The listing builds one solid part. Answer for the finished solid, in the listing's coordinates (mm). Round coordinates to 2 decimals unless told otherwise and drop trailing zeros. Order: outer loops, then holes, each group sorted by start corner. A loop starts at its lowest first (then second) coordinate and runs counter-clockwise, first axis right, second up. Notation, with made-up numbers: (-2, 81.25) -> (5, 81.25) arc R28 ccw to (5, 115.25) -> close; hole circle Ø4 at (38.25, 29). An arc over 180 degrees is marked (long way). Return JSON: item names as keys, results as strings. Group by question number.
(1) The part is cut by section D-D (x = -28.5). Determine the outline of the cut face in (y, z), plus the area to 3 significant figures.
(2) The part is cut by section A-A (y = 0). Determine the outline of the cut face in (x, z) (3 decimals), plus the area to 3 significant figures.
(3) The part is cut by section C-C (z = 10). Determine the outline of the cut face in (x, y), plus the area to 3 significant figures.
(4) Consider line 1 (Y direction, x = 0, z = 12.5); line 2 (Z direction, x = 29, y = 0); line 3 (Y direction, x = 10, z = 16). Determine where each line is inside the solid, lowest interval first. Write a range as [from, to].
(5) Determine the mould class of faces 1 (the face through (-8, 23, 6.35)), 2 (the face through (23.016, 7.248, 14.568)), 3 (the face through (-3.887, -17.503, 23.168)) for opening direction X: +X half, -X half, draft (parallel to the pull), parting line (faces both ways), or undercut.
(6) Each of these flat-tipped pins is pushed along its axis until it touches: pin 1 (1.5 mm diameter, centred on x = -25, z = 13, fed in from -Y); pin 2 (12 mm diameter, centred on y = 16, z = 14, fed in from -X); pin 3 (4 mm diameter, centred on x = 24.5, y = -7.5, fed in from +Z); pin 4 (1.5 mm diameter, centred on x = -8, z = 10.5, fed in from +Y). Where does it stop, or does it pass through?
from build123d import *

# Parameters (mm, degrees)
F0_R     = 24.13
F0_R_2   = 17.78
F1_DEPTH = 25.4
F2_R     = 33.655
F2_R_2   = 24.13
F3_DEPTH = 6.35
F4_SIZE  = 2.38125


with BuildPart() as f1:
    # F0 (on Top) → F1 (new body)
    with BuildSketch(Plane.XY):
        Circle(F0_R)
        Circle(F0_R_2, mode=Mode.SUBTRACT)
    extrude(amount=F1_DEPTH)

    # F2 (on Top) → F3 (join)
    with BuildSketch(Plane.XY):
        Circle(F2_R)
        Circle(F2_R_2, mode=Mode.SUBTRACT)
    extrude(amount=F3_DEPTH)

    # F4
    f4_edges = [f1.edges().sort_by_distance(p)[0] for p in [
        (-24.13, 0, 25.4),
        (-17.78, 0, 25.4),
    ]]
    chamfer(f4_edges, length=F4_SIZE)


solid = f1.part
Answer below:
{
 "1": {"outline": "(-17.9, 0) -> (17.9, 0) -> (17.9, 6.35) -> (-17.9, 6.35) -> close", "area": "227 mm²"},
 "2": {"outline": "(-33.655, 0) -> (-17.78, 0) -> (-17.78, 23.019) -> (-20.161, 25.4) -> (-21.749, 25.4) -> (-24.13, 23.019) -> (-24.13, 6.35) -> (-33.655, 6.35) -> close; (17.78, 0) -> (33.655, 0) -> (33.655, 6.35) -> (24.13, 6.35) -> (24.13, 23.019) -> (21.749, 25.4) -> (20.161, 25.4) -> (17.78, 23.019) -> close", "area": "432 mm²"},
 "3": {"outline": "circle Ø48.26 at (0, 0); hole circle Ø35.56 at (0, 0)", "area": "836 mm²"},
 "4": {"line 1": "y = [-24.13, -17.78], [17.78, 24.13]", "line 2": "z = [0, 6.35]", "line 3": "y = [-21.96, -14.7], [14.7, 21.96]"},
 "5": {"face 1": "draft", "face 2": "parting line", "face 3": "undercut"},
 "6": {"pin 1": "passes through", "pin 2": "stops at x = -21.96", "pin 3": "stops at z = 23.53", "pin 4": "stops at y = 23.02"}
}
